from build123d import *

# Parameters (mm, degrees)
BOSS_EXTRUDE1_DEPTH     = 210
CUT_EXTRUDE1_DEPTH      = 60
FILLET1_R               = 10
FILLET2_R               = 10
SKETCH3_R               = 50
BOSS_EXTRUDE2_DEPTH     = 5
CUT_EXTRUDE2_DEPTH      = 452.914312828
CUT_EXTRUDE2_DEPTH_BACK = 452.914312828
SKETCH4_W               = 303.312029478
SKETCH4_H               = 103.575222475


with BuildPart() as part:
    # Sketch1 → Boss-Extrude1 (new body)
    with BuildSketch(Plane(origin=(0, 0, 0), x_dir=(1, 0, 0), z_dir=(0, 1, 0))):
        Polygon((-177.169811321, 160.999367101), (-137.169811321, 160.999367101), (-87.169811321, 154.961631252), (108.540145677, 113.759535042), (136.34102955, 85), (366.34102955, 85), (366.34102955, -85), (136.34102955, -85), (108.540145677, -113.759535042), (-87.169811321, -154.961631252), (-137.169811321, -160.999367101), (-177.169811321, -160.999367101), align=None)
    extrude(amount=BOSS_EXTRUDE1_DEPTH)

    # Sketch2 → Cut-Extrude1 (cut)
    with BuildSketch(Plane.XY.offset(160)):
        Polygon((-177.169811321, 0), (366.34102955, 145), (366.34102955, 0), align=None)
    extrude(amount=-CUT_EXTRUDE1_DEPTH, mode=Mode.SUBTRACT)

    # Fillet1
    # the kernel refuses this fillet: 10 mm, written as the material it adds along each edge
    with BuildSketch(Plane(origin=(136.34102955, 0, 85), x_dir=(-0.6950220968474797, 0, 0.7189883760491075), z_dir=(0, 1, 0))) as fillet1_piece_1:
        with BuildLine():
            CenterArc((FILLET1_R * 0.424176403002, FILLET1_R), FILLET1_R, 224.028978069, 45.971021931)
            Line((-FILLET1_R * 0.294811973047, FILLET1_R * 0.304977903153), (0, 0))
            Line((0, 0), (FILLET1_R * 0.424176403002, 0))
        make_face()
    extrude(amount=210)
    # the kernel refuses this fillet: 10 mm, written as the material it takes off along each edge
    with BuildSketch(Plane(origin=(108.540145677, 68.559927222, 113.759535042), x_dir=(0.6950220968474767, 0, -0.7189883760491101), z_dir=(0, 1, 0))) as fillet1_2_piece_1:
        with BuildLine():
            CenterArc((FILLET1_R * 0.306516798333, FILLET1_R), FILLET1_R, 235.917636109, 34.082363891)
            Line((-FILLET1_R * 0.253867285946, FILLET1_R * 0.17176713535), (0, 0))
            Line((0, 0), (FILLET1_R * 0.306516798333, 0))
        make_face()
    extrude(amount=149.102992736, mode=Mode.SUBTRACT)
    with BuildSketch(Plane(origin=(-87.169811321, 22.918324442, 154.961631252), x_dir=(0.9785497849867442, 0, -0.20601048104986486), z_dir=(0, 1, 0))) as fillet1_2_piece_2:
        with BuildLine():
            CenterArc((FILLET1_R * 0.0436894476987, FILLET1_R), FILLET1_R, 264.996739811, 5.003260189)
            Line((-FILLET1_R * 0.0435229794225, FILLET1_R * 0.00381026277338), (0, 0))
            Line((0, 0), (FILLET1_R * 0.0436894476986, 0))
        make_face()
    extrude(amount=188.173911751, mode=Mode.SUBTRACT)
    with BuildSketch(Plane(origin=(-137.169811321, -1.50397119, 160.999367101), x_dir=(-1, 0, 0), z_dir=(0, 1, 0))) as fillet1_2_piece_3:
        with BuildLine():
            CenterArc((FILLET1_R * 0.0601588475808, -FILLET1_R), FILLET1_R, 90, 6.88539785)
            Line((-FILLET1_R * 0.0597249775946, -FILLET1_R * 0.00721207276614), (0, 0))
            Line((0, 0), (FILLET1_R * 0.0601588475808, 0))
        make_face()
    extrude(amount=213.007942379, mode=Mode.SUBTRACT)

    # Fillet2
    # the kernel refuses this fillet: 10 mm, written as the material it adds along each edge
    with BuildSketch(Plane(origin=(136.34102955, 0, -85), x_dir=(-0.695022096847478, 0, -0.7189883760491093), z_dir=(0, 1, 0))) as fillet2_piece_1:
        with BuildLine():
            CenterArc((FILLET2_R * 0.424176403002, -FILLET2_R), FILLET2_R, 90, 45.971021931)
            Line((-FILLET2_R * 0.294811973047, -FILLET2_R * 0.304977903153), (0, 0))
            Line((0, 0), (FILLET2_R * 0.424176403002, 0))
        make_face()
    extrude(amount=210)
    # the kernel refuses this fillet: 10 mm, written as the material it takes off along each edge
    with BuildSketch(Plane(origin=(-137.169811321, -1.50397119, -160.999367101), x_dir=(-1, 0, 0), z_dir=(0, 1, 0))) as fillet2_2_piece_1:
        with BuildLine():
            CenterArc((FILLET2_R * 0.0601588475808, FILLET2_R), FILLET2_R, 263.11460215, 6.88539785)
            Line((-FILLET2_R * 0.0597249775946, FILLET2_R * 0.00721207276614), (0, 0))
            Line((0, 0), (FILLET2_R * 0.0601588475808, 0))
        make_face()
    extrude(amount=213.007942379, mode=Mode.SUBTRACT)
    with BuildSketch(Plane(origin=(-87.169811321, -1.092236192, -154.961631252), x_dir=(-0.9927879272338658, 0, -0.11988382517539375), z_dir=(0, 1, 0))) as fillet2_2_piece_2:
        with BuildLine():
            CenterArc((FILLET2_R * 0.0436894476987, FILLET2_R), FILLET2_R, 264.996739811, 5.003260189)
            Line((-FILLET2_R * 0.0435229794225, FILLET2_R * 0.00381026277338), (0, 0))
            Line((0, 0), (FILLET2_R * 0.0436894476986, 0))
        make_face()
    extrude(amount=212.184472385, mode=Mode.SUBTRACT)
    with BuildSketch(Plane(origin=(108.540145677, -7.662919958, -113.759535042), x_dir=(-0.9785497849867494, 0, -0.20601048104984027), z_dir=(0, 1, 0))) as fillet2_2_piece_3:
        with BuildLine():
            CenterArc((FILLET2_R * 0.306516798333, FILLET2_R), FILLET2_R, 235.917636109, 34.082363891)
            Line((-FILLET2_R * 0.253867285946, FILLET2_R * 0.17176713535), (0, 0))
            Line((0, 0), (FILLET2_R * 0.306516798333, 0))
        make_face()
    extrude(amount=225.325839917, mode=Mode.SUBTRACT)

    # Sketch3 → Boss-Extrude2 (add)
    with BuildSketch(Plane.XZ):
        with Locations(Location((312.605658758, 0, 0), (0, 0, 270))):
            Circle(SKETCH3_R)
    extrude(amount=BOSS_EXTRUDE2_DEPTH)

    # Sketch4 → Cut-Extrude2 (cut, two sides: drawn at the far end of the back side and taken through both)
    with BuildSketch(Plane.XZ.offset(-CUT_EXTRUDE2_DEPTH_BACK)):
        with Locations((-25.513796582, 151.787611238)):
            Rectangle(SKETCH4_W, SKETCH4_H)
    extrude(amount=CUT_EXTRUDE2_DEPTH + CUT_EXTRUDE2_DEPTH_BACK, mode=Mode.SUBTRACT)


solid = part.part
Geometry: final body of the model. Coordinates: model frame, mm. A direction names the side the tool comes from. Give positions to 0.01 mm unless a question says otherwise; leave off trailing zeros. Loops run counter-clockwise (first coordinate to the right, second up) from the corner with the lowest first, then second, coordinate; pieces in that order, holes last. Notation, with made-up numbers: M 69.5,85.25 L 82.5,85.25 A29 cw 82.5,114.25 Z; hole C 20,-3 d11. An arc over 180 degrees is marked long. Put each result on its own line as item: value. Start each with the question number.
1) Cut plane D-D (z = 41). Output: boundary loops of the cut face in (x, y).
2) Cut plane B-B (y = 41). Output: boundary loops of the cut face in (x, z), then the cut area to 3 significant figures.
3) Contact query for flat-ended pins moving along their axis: pin 1 (10 mm diameter, centred on x = 197.5, y = 99, fed in from +Z); pin 2 (6 mm diameter, centred on x = -9.5, y = 150.5, fed in from -Z); pin 3 (2 mm diameter, centred on x = -10, z = 30, fed in from -Y). Output: stop coordinate, or through.
4) Ray query, line 1 along Y through (x, z) = (-15, -48); line 2 along Z through (x, y) = (316.5, 86); line 3 along X through (y, z) = (152, -94). Return the intervals inside material, ascending.
5) Access query for faces 1 (the flat face through (252, 104, -85)), 2 (the cylindrical face through (362.18, -2.46, 6.51)), 3 (the flat face through (255, 104, 85)). Directions: +Z, -Z, +X, -X, +Y, -Y. A direction counts if a zero-diameter tool reaches every point of the face in a straight line with its end or side. Return the directions, or none.
6) Cut plane A-A (z = 0). Output: boundary loops of the cut face in (x, y).
7) Cut plane C-C (x = 250). Output: boundary loops of the cut face in (y, z), then the cut area to 3 significant figures.
Verdict:
1. outline: M -177.17,0 L 283.99,0 L 283.99,-5 L 341.22,-5 L 341.22,0 L 366.34,0 L 366.34,210 L -177.17,210 Z
2. outline: M -177.17,-161 L -137.77,-161 A10 ccw -136.57,-160.93 L -87.6,-155.01 A10 ccw -86.74,-154.87 L 105.54,-114.39 A10 ccw 110.67,-111.56 L 133.39,-88.05 A10 cw 140.58,-85 L 366.34,-85 L 366.34,85 L 140.58,85 A10 cw 133.39,88.05 L 121.84,100 L -177.17,100 Z
2. area: 114,000 mm2
3. pin 1: z = 85
3. pin 2: z = -139.24
3. pin 3: y = 0
4. line 1: 0 to 210
4. line 2: -85 to 85
4. line 3: -177.17 to 127.64
5. face 1: -Z, +X, +Y, -Y
5. face 2: -Y
5. face 3: +Z, +X, +Y, -Y
6. outline: M -177.17,0 L 262.61,0 L 262.61,-5 L 362.61,-5 L 362.61,0 L 366.34,0 L 366.34,210 L -177.17,210 Z
7. outline: M 0,-85 L 210,-85 L 210,85 L 0,85 Z
7. area: 35,700 mm2
